Autodesk Inventor part; units mm, degrees
ref_plane "YZ Plane" through (0, 0, 0) normal (1, 0, 0) x (0, 1, 0)
ref_plane "XZ Plane" through (0, 0, 0) normal (0, 1, 0) x (-1, 0, 0)
ref_plane "XY Plane" through (0, 0, 0) normal (0, 0, 1) x (1, 0, 0)
sketch "Sketch1" plane through (0, 0, 0) normal (0, 0, 1) x (1, 0, 0)
  circle A0 centre (0, 0) radius 12.5
  dimension "d0" = 25
extrude "Extrusion1" add sketch "Sketch1" along normal blind 25
sketch "Sketch2" plane through (0, 0, 0) normal (1, 0, 0) x (0, 1, 0)
  line L0 (0, 0) -> (0, 24.8569) construction
  line L1 (12.5, 0) -> (12.5, 25)
  line L2 (12.5, 23.85) -> (4.58, 23.85)
  line L3 (4.58, 23.85) -> (4.58, 21.6)
  line L4 (4.58, 21.6) -> (12.5, 21.6)
  line L5 (12.5, 21.6) -> (12.5, 23.85)
  line L6 (12.5, 25) -> (-12.5, 25)
  line L7 (12.5, 20.45) -> (4.58, 20.45)
  line L8 (4.58, 20.45) -> (4.58, 18.2)
  line L9 (4.58, 18.2) -> (12.5, 18.2)
  line L10 (12.5, 18.2) -> (12.5, 20.45)
  line L11 (12.5, 17.05) -> (4.58, 17.05)
  line L12 (4.58, 17.05) -> (4.58, 14.8)
  line L13 (4.58, 14.8) -> (12.5, 14.8)
  line L14 (12.5, 14.8) -> (12.5, 17.05)
  line L15 (12.5, 13.65) -> (4.58, 13.65)
  line L16 (4.58, 13.65) -> (4.58, 11.4)
  line L17 (4.58, 11.4) -> (12.5, 11.4)
  line L18 (12.5, 11.4) -> (12.5, 13.65)
  line L19 (12.5, 10.25) -> (4.58, 10.25)
  line L20 (4.58, 10.25) -> (4.58, 8)
  line L21 (4.58, 8) -> (12.5, 8)
  line L22 (12.5, 8) -> (12.5, 10.25)
  line L23 (12.5, 6.85) -> (4.58, 6.85)
  line L24 (4.58, 6.85) -> (4.58, 4.6)
  line L25 (4.58, 4.6) -> (12.5, 4.6)
  line L26 (12.5, 4.6) -> (12.5, 6.85)
  line L27 (12.5, 3.45) -> (4.58, 3.45)
  line L28 (4.58, 3.45) -> (4.58, 1.2)
  line L29 (4.58, 1.2) -> (12.5, 1.2)
  line L30 (12.5, 1.2) -> (12.5, 3.45)
  dimension "d3" = 2.25
  dimension "d4" = 1.15
  dimension "d5" = 7.92
  dimension "d8" = 3.4
revolve "Revolution1" cut sketch "Sketch2" angle 360 about axis through (0, 0, 0) along (0, 0, 1)
sketch "Sketch3" plane through (0, 0, 25) normal (0, 0, 1) x (1, 0, 0)
  circle A0 centre (0, 0) radius 2.46
  dimension "d14" = 4.92
extrude "Extrusion2" cut sketch "Sketch3" against normal through all
thread "Thread1"
chamfer "Chamfer1" distance 0.25 angle 45 1 edges at (-2.46, 0, 25)
chamfer "Chamfer2" distance 0.25 angle 45 1 edges at (-2.46, 0, 0)
properties part number "Cooling fin" material "Aluminum 5005-H18"
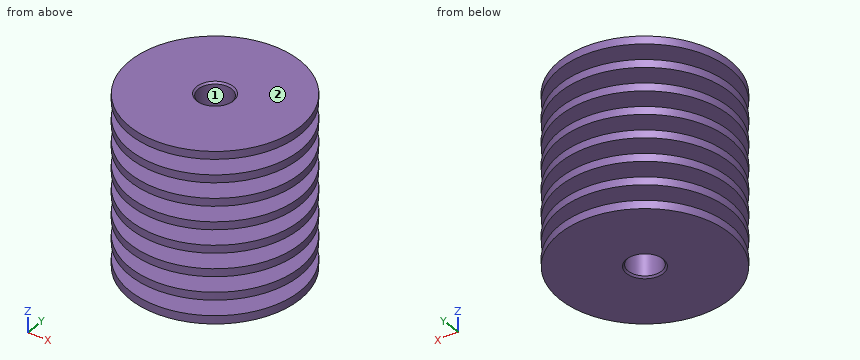
Can you work these out from the model? Positions are in its coordinate system, mm. Face numbers are marked on the shaded views. Round coordinates to 2 decimals unless told otherwise and drop trailing zeros. Loops run counter-clockwise (first coordinate to the right, second up) from the corner with the lowest first, then second, coordinate; pieces in that order, holes last. Notation, with made-up numbers: M -9,-16 L 11,-16 A24 cw 11,9 Z; hole C 45,42 d9. An arc over 180 degrees is marked long. Answer as a JSON object with one key per item and string values. Group by question number.
Q1. Imagine slicing it at C-C, the plane z = 9.25. Please give me the cut outline in (x, y), then the cut area to 3 significant figures.
Q2. Please list where these lines run through material, in increasing order: L1, parallel to Y at x = 0, z = 7.25; L2, parallel to Y at x = 0, z = 18.5; L3, parallel to Z at x = -2.25, y = -1.5.
Q3. Imagine slicing it at A-A, the plane y = -7.5. Count the separate pieces of the cut face and the enclosed holes in it, then the cut area to 3 significant figures.
Q4. We'd pull the mould along Y, two halves only. Please class the marked faces 1 and 2: +Y half, -Y half, draft (parallel to the pull), parting line (faces both ways), or undercut.
Q5. Will these pins go through, and if not, where does the flat tip stop? pin 1 (12.5 mm diameter, centred on x = 1.5, y = -1.5, fed in from -Z); pin 2 (2 mm diameter, centred on x = -9, z = 19, fed in from -Y); pin 3 (6 mm diameter, centred on x = -5, z = 18.5, fed in from -Y); pin 4 (6 mm diameter, centred on x = -3.5, z = 14.5, fed in from -Y).
Findings:
{
 "1": {"outline": "C 0,0 d9.16; hole C 0,0 d4.92", "area": "46.9 mm2"},
 "2": {"L1": "y = -12.5 to -2.46, 2.46 to 12.5", "L2": "y = -4.58 to -2.46, 2.46 to 4.58", "L3": "z = 0.01 to 24.99"},
 "3": {"separate pieces": "8", "enclosed holes": "0", "area": "185 mm2"},
 "4": {"face 1": "undercut", "face 2": "draft"},
 "5": {"pin 1": "stops at z = 0", "pin 2": "stops at y = -9.26", "pin 3": "stops at y = -12.34", "pin 4": "stops at y = -12.49"}
}
